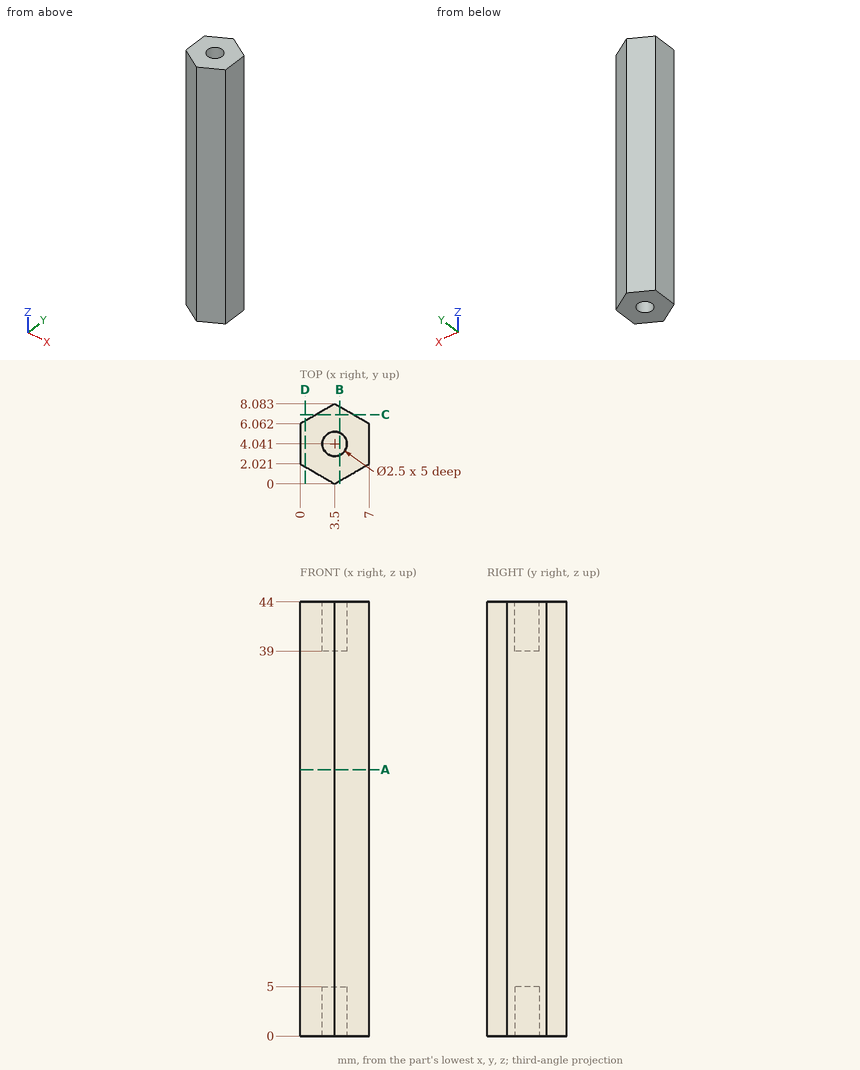
Here's the drawing with two shaded views (mm, measured from the low corner). I have some questions. Coordinates: 2 decimals unless noted, no trailing zeros. Loops run counter-clockwise (first coordinate to the right, second up) from the corner with the lowest first, then second, coordinate; pieces in that order, holes last. Notation, with made-up numbers: M 70.5,27 L 74.5,27 A17 ccw 74.5,54 Z; hole C -1,65.25 d2. An arc over 180 degrees is marked long. Put each result on its own line as item: value. Start each with the question number.
(1) I need wall thicknesses on probe 1 along Y at (x, z) = (3.5, 1.4); probe 2 along Z at (x, y) = (4, 4.5); probe 3 along X at (y, z) = (6.5, 31) (1 decimal). Which ranges of each line are inside material? Lowest first, please.
(2) Imagine slicing it at D-D on x = 0.5. List the corners of the cut face in (y, z) for me.
(3) Imagine slicing it at A-A on z = 27. List the corners of the cut face in (x, y) for me.
(4) Imagine slicing it at C-C on y = 7. List the corners of the cut face in (x, z) for me (1 decimal).
(5) Imagine slicing it at B-B on x = 4. List the corners of the cut face in (y, z) for me (1 decimal).
(6) Will these pins go through, and if not, where does the flat tip stop? pin 1 Ø0.8 at (x, y) = (3.5, 4) entering from +Z; pin 2 Ø1.5 at (x, y) = (3.5, 4.04) entering from -Z.
Worked answers:
1. probe 1: y = 0 to 2.79, 5.29 to 8.08
1. probe 2: z = 5 to 39
1. probe 3: x = 0.8 to 6.2
2. outline: M 1.73,0 L 6.35,0 L 6.35,44 L 1.73,44 Z
3. outline: M 0,2.02 L 3.5,0 L 7,2.02 L 7,6.06 L 3.5,8.08 L 0,6.06 Z
4. outline: M 1.6,0 L 5.4,0 L 5.4,44 L 1.6,44 Z
5. outline: M 0.3,0 L 2.9,0 L 2.9,5 L 5.2,5 L 5.2,0 L 7.8,0 L 7.8,44 L 5.2,44 L 5.2,39 L 2.9,39 L 2.9,44 L 0.3,44 Z
6. pin 1: stops at z = 39
6. pin 2: stops at z = 5
